CAD build for the part. Positions are in the model's coordinates, mm. Face numbers are marked on the shaded views. Coordinates: 2 decimals unless noted, no trailing zeros. Order: outer loops, then holes, each group sorted by start corner. A loop starts at its lowest first (then second) coordinate and runs counter-clockwise, first axis right, second up. Notation, with made-up numbers: M 9,-16 L 57,-16 A29 ccw 57,9 Z; hole C 72.25,-35 d10. An arc over 180 degrees is marked long. Write item = value, one per line.
from build123d import *

# Parameters (mm, degrees)
F0_W     = 127
F0_H     = 127
F0_R     = 37.719
F1_DEPTH = 12.7
F2_SIZE2 = 6.35
F2_SIZE  = 6.35


with BuildPart() as f1:
    # F0 (on Front) → F1 (new body)
    with BuildSketch(Plane.XZ):
        Rectangle(F0_W, F0_H)
        Circle(F0_R, mode=Mode.SUBTRACT)
    extrude(amount=F1_DEPTH)

    # F2
    f2_edges = [f1.edges().sort_by_distance(p)[0] for p in [
        (-37.719, 0, 0),
    ]]
    chamfer(f2_edges, length=F2_SIZE, length2=F2_SIZE2)


solid = f1.part
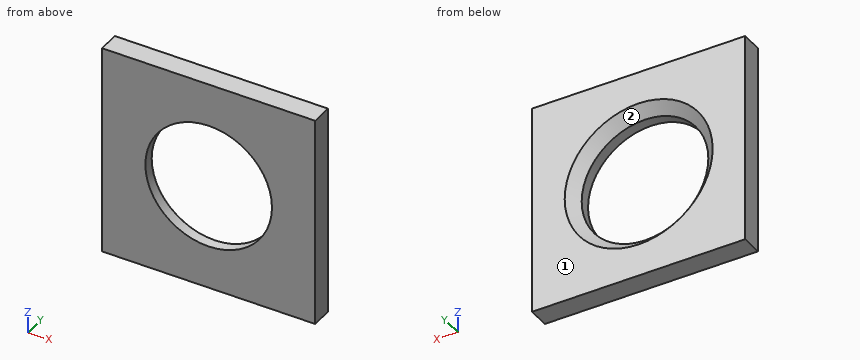
(1) Pull direction Z, two halves, no side cores. Call the marked faces 1 and 2: +Z half, -Z half, draft (parallel to the pull), parting line (faces both ways), or undercut.
Evaluation:
face_1 = draft
face_2 = undercut
(2) Slice it at C-C, the plane y = -8.5. Write the cut outline in (x, z), then the cut area to 3 significant figures.
Evaluation:
outline = M -63.5,-63.5 L 63.5,-63.5 L 63.5,63.5 L -63.5,63.5 Z; hole C 0,0 d75.44
area = 11,700 mm²
(3) Wall check: line 1 (Z direction, x = 0, y = -10.25); line 2 (X direction, y = -4, z = -7.5); line 3 (Z direction, x = 30, y = -7.5). Give the ranges that are in metal, low to high. Write a range as from..to.
Evaluation:
line_1 = -63.5..-37.72, 37.72..63.5
line_2 = -63.5..-39.36, 39.36..63.5
line_3 = -63.5..-22.86, 22.86..63.5
(4) Slice it at A-A, the plane x = 0. Write the cut outline in (y, z), then the cut area to 3 significant figures.
Evaluation:
outline = M -12.7,-63.5 L 0,-63.5 L 0,-44.07 L -6.35,-37.72 L -12.7,-37.72 Z; M -12.7,37.72 L -6.35,37.72 L 0,44.07 L 0,63.5 L -12.7,63.5 Z
area = 615 mm²
(5) Slice it at B-B, the plane z = 0. Write the cut outline in (x, y), then the cut area to 3 significant figures.
Evaluation:
outline = M -63.5,-12.7 L -37.72,-12.7 L -37.72,-6.35 L -44.07,0 L -63.5,0 Z; M 37.72,-12.7 L 63.5,-12.7 L 63.5,0 L 44.07,0 L 37.72,-6.35 Z
area = 615 mm²
